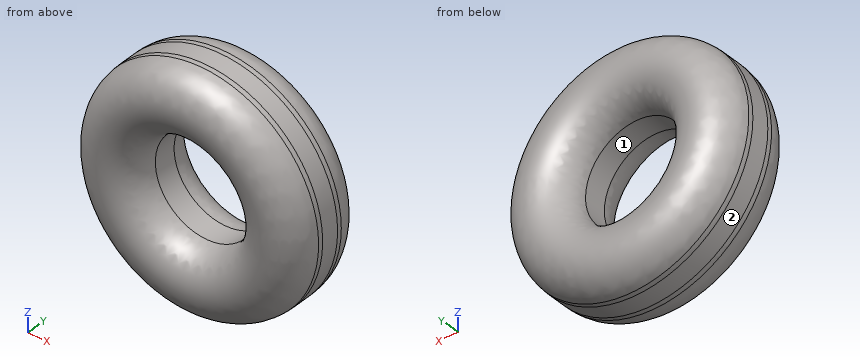
```python
from build123d import *

# Parameters (mm, degrees)
F0_R     = 25.4
F1_DEPTH = 32.45895
F2_R     = 14.232827062
F3_R     = 11.0557662792
F4_DEPTH = 97.05153
F5_R     = 7.1628


with BuildPart() as f1:
    # F0 (on Front) → F1 (new body)
    with BuildSketch(Plane.XZ):
        Circle(F0_R)
    extrude(amount=F1_DEPTH)

    # F2
    f2_edges = [f1.edges().sort_by_distance(p)[0] for p in [
        (-25.4, -32.45895, 0),
        (-25.4, 0, 0),
    ]]
    fillet(f2_edges, radius=F2_R)

    # F3 (on Front) → F4 (cut)
    with BuildSketch(Plane.XZ):
        Circle(F3_R)
    extrude(amount=F4_DEPTH, mode=Mode.SUBTRACT)

    # F5
    f5_edges = [f1.edges().sort_by_distance(p)[0] for p in [
        (-11.055766, 0, 0),
        (11.055766, -16.229475, 0),
        (-11.055766, -32.45895, 0),
    ]]
    fillet(f5_edges, radius=F5_R)


solid = f1.part
```
The model under review builds one solid part; all positions refer to its coordinate system, in mm. Face numbers are marked on the shaded views. Give positions to 0.01 mm unless a question says otherwise; leave off trailing zeros. Write each loop counter-clockwise with the first axis right and the second up, starting at its lowest first coordinate (ties: lowest second). Pieces come first, ordered by that corner, then holes. Notation, with made-up numbers: M -14.75,8.25 L 44.25,8.25 A12 ccw 44.25,29.25 Z; hole C 70,30.5 d8. An arc over 180 degrees is marked long. Write item = value, one per line. Start each with the question number.
Q1. Clearance check with flat-ended pins moving along their axes: pin 1 (3 mm diameter, centred on x = -17.5, y = -21, fed in from -Z); pin 2 (1 mm diameter, centred on x = 13, y = -16.5, fed in from +Z); pin 3 (10 mm diameter, centred on x = -4.5, y = -16.5, fed in from +Z). State where each tip first meets the part, or that it passes through.
Q2. Mouldability with a two-part tool opening along X and no side actions: class the marked faces 1 and 2 as released by +X, released by -X, zero draft, split by the parting line, or undercut.
Q3. For line 1 (Z direction, x = 0, y = -16.5); line 2 (X direction, y = -19.25, z = 0); line 3 (X direction, y = -16, z = 10), list the stretches that pass through material, from the lowest coordinate up.
Q4. We need section A-A (y = -15). State the section outline as (x, z) points.
Result set:
q1.pin_1 = -19.35
q1.pin_2 = 22.11
q1.pin_3 = 25.4
q2.face_1 = undercut
q2.face_2 = split by the parting line
q3.line_1 = -25.4 to -11.06, 11.06 to 25.4
q3.line_2 = -25.36 to -11.07, 11.07 to 25.36
q3.line_3 = -23.35 to -4.71, 4.71 to 23.35
q4.outline = C 0,0 d50.8; hole C 0,0 d22.11
